Work out the finished part from the listing and answer in its coordinate system (mm). Round coordinates to 2 decimals unless told otherwise and drop trailing zeros. Write each loop counter-clockwise with the first axis right and the second up, starting at its lowest first coordinate (ties: lowest second). Pieces come first, ordered by that corner, then holes.
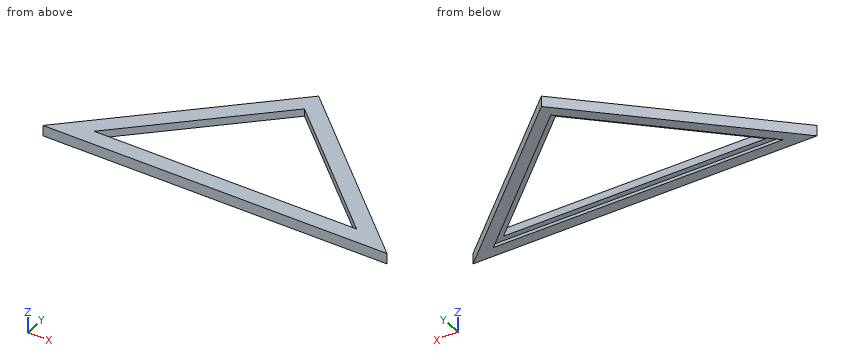
from build123d import *

# Parameters (mm, degrees)
SALIENTE_EXTRUIR1_DEPTH = 10
CORTAR_EXTRUIR1_DEPTH   = 3


with BuildPart() as part:
    # Croquis1 → Saliente-Extruir1 (new body)
    with BuildSketch(Plane.XY):
        Polygon((0, 0), (320, 0), (160, 150), align=None)
        Polygon((160, 129.439019813), (282.068287801, 15), (37.931712199, 15), align=None, mode=Mode.SUBTRACT)
    extrude(amount=SALIENTE_EXTRUIR1_DEPTH)

    # Croquis2 → Cortar-Extruir1 (cut)
    with BuildSketch(Plane(origin=(0, 0, 0), x_dir=(-1, 0, 0), z_dir=(0, 0, -1))):
        Polygon((-294.712191867, 10), (-25.287808133, 10), (-160, 136.292679875), align=None)
    extrude(amount=-CORTAR_EXTRUIR1_DEPTH, mode=Mode.SUBTRACT)


solid = part.part
Q1. Given pin 1 (0.9 mm diameter, centred on x = 189.5, z = 2, fed in from +Y); pin 2 (2 mm diameter, centred on y = 74, z = 5, fed in from -X); pin 3 (1 mm diameter, centred on x = 116.5, y = 86.5, fed in from +Z); pin 4 (3 mm diameter, centred on y = 25, z = 8, fed in from +X), each flat-ended and moving along its own axis, determine where each tip first touches the part or whether it passes through.
Q2. Find section B-B (x = 154.5). Determine the outline of the cut face in (y, z), plus the area to 3 significant figures.
Q3. Find section C-C (z = 8). Determine the outline of the cut face in (x, y), plus the area to 3 significant figures.
Q4. Find section A-A (y = 20). Determine the outline of the cut face in (x, z).
Q5. Find the intervals of material crossed by L1, parallel to Y at x = 220, z = 4.25; L2, parallel to X at y = 16, z = 2.5; L3, parallel to Y at x = 126, z = 2.75 (3 decimals), in increasing order.
Q6. Find section D-D (x = 291). Determine the outline of the cut face in (y, z), plus the area to 3 significant figures.
Report:
1. pin 1: stops at y = 122.77
1. pin 2: stops at x = 77.87
1. pin 3: passes through
1. pin 4: stops at x = 294.93
2. outline: (0, 0) - (10, 0) - (10, 3) - (15, 3) - (15, 10) - (0, 10) - close; (124.28, 3) - (131.14, 3) - (131.14, 0) - (144.84, 0) - (144.84, 10) - (124.28, 10) - close
2. area: 320 mm2
3. outline: (0, 0) - (320, 0) - (160, 150) - close; hole (37.93, 15) - (282.07, 15) - (160, 129.44) - close
3. area: 10,000 mm2
4. outline: (21.33, 0) - (35.95, 0) - (35.95, 3) - (43.27, 3) - (43.27, 10) - (21.33, 10) - close; (276.73, 3) - (284.05, 3) - (284.05, 0) - (298.67, 0) - (298.67, 10) - (276.73, 10) - close
5. L1: y = 0 to 15, 73.19 to 93.75
5. L2: x = 17.07 to 31.69, 288.31 to 302.93
5. L3: y = 0 to 10, 104.418 to 118.125
6. outline: (0, 0) - (10, 0) - (10, 3) - (13.48, 3) - (13.48, 0) - (27.19, 0) - (27.19, 10) - (0, 10) - close
6. area: 261 mm2
